For this review, take the finished solid that the model builds, in its own axes (mm). A direction names the side the tool comes from. Coordinates: 2 decimals unless noted, no trailing zeros. Write each loop counter-clockwise with the first axis right and the second up, starting at its lowest first coordinate (ties: lowest second). Pieces come first, ordered by that corner, then holes.
Autodesk Inventor part; units mm, degrees
ref_plane "YZ Plane" through (0, 0, 0) normal (1, 0, 0) x (0, 1, 0)
ref_plane "XZ Plane" through (0, 0, 0) normal (0, 1, 0) x (-1, 0, 0)
ref_plane "XY Plane" through (0, 0, 0) normal (0, 0, 1) x (1, 0, 0)
sketch "Sketch1" plane through (0, 0, 0) normal (0, 0, 1) x (1, 0, 0)
  line L0 (-12.7, 0) -> (12.7, 0) construction
  line L1 (12.7, 0) -> (12.7, -57.15)
  line L2 (12.7, -57.15) -> (-12.7, -57.15)
  line L3 (-12.7, -57.15) -> (-12.7, 0) construction
  line L4 (-35.1269, 0) -> (-12.7, -11.9246) construction
  line L5 (-12.7, -11.9246) -> (-36.5492, -56.7783)
  line L6 (-36.5492, -56.7783) -> (-58.976, -44.8537)
  line L7 (-58.976, -44.8537) -> (-35.1269, 0)
  line L8 (-23.9134, -5.9623) -> (-47.7626, -50.816) construction
  line L9 (-35.1269, 0) -> (12.7, 0)
  line L10 (-12.7, -11.9246) -> (-12.7, -57.15)
  point P0 (0, 0)
  point P1 (0, 0)
  point P2 (-29.8757, -17.1757)
  point P3 (-41.8003, -39.6026)
  point P4 (0, -12.7)
  point P5 (0, -38.1)
  dimension "d0" = 25.4
  dimension "d1" = 25.4
  dimension "d2" = 28
  dimension "d3" = 50.8
  dimension "d4" = 25.4
  dimension "d5" = 12.7
  dimension "d6" = 25.4
  dimension "d7" = 12.7
  dimension "d8" = 57.15
extrude "Extrusion1" add sketch "Sketch1" against normal blind 6.35
hole "Hole1" at (-29.8757, -17.1757, 0) at (-41.8003, -39.6026, 0) at (0, -12.7, 0) at (0, -38.1, 0) direction (0, 0, -1) diameter 5.1054 end through all
sketch "Sketch2" plane through (0, 0, 0) normal (0, 0, 1) x (1, 0, 0)
  circle A0 centre (0, -12.7) radius 2.5527 construction
  circle A1 centre (-29.8757, -17.1757) radius 2.5527 construction
  circle A2 centre (-41.8003, -39.6026) radius 2.5527 construction
  circle A3 centre (0, -38.1) radius 2.5527 construction
  line L0 (-12.7, -57.15) -> (12.7, -57.15) construction
  line L1 (12.7, -57.15) -> (12.7, 0) construction
  line L2 (12.7, 0) -> (-35.1269, 0)
  line L3 (-35.1269, 0) -> (-58.976, -44.8537) construction
  line L4 (-58.976, -44.8537) -> (-36.5492, -56.7783) construction
  line L5 (-36.5492, -56.7783) -> (-12.7, -11.9246) construction
  line L6 (-12.7, -11.9246) -> (-12.7, -57.15) construction
  circle A4 centre (0, -12.7) radius 2.5527 construction
  circle A5 centre (-29.8757, -17.1757) radius 2.5527 construction
  circle A6 centre (-41.8003, -39.6026) radius 2.5527 construction
  circle A7 centre (0, -38.1) radius 2.5527 construction
  line L7 (12.7, 0) -> (12.7, -57.15) construction
  line L8 (12.7, -57.15) -> (-12.7, -57.15) construction
  line L9 (-12.7, -57.15) -> (-12.7, -11.9246) construction
  line L10 (-36.5492, -56.7783) -> (-58.976, -44.8537) construction
  line L11 (-58.976, -44.8537) -> (-35.1269, 0) construction
  line L12 (-35.1269, 0) -> (12.7, 0) construction
  circle A8 centre (-11.2134, 101.6) radius 14.2875 construction
  line L13 (12.7, 0) -> (-35.1269, 0) construction
  line L14 (-35.1269, 0) -> (-58.976, -44.8537) construction
  circle A9 centre (0, -12.7) radius 2.5527 construction
  circle A10 centre (-29.8757, -17.1757) radius 2.5527 construction
  circle A11 centre (-41.8003, -39.6026) radius 2.5527 construction
  circle A12 centre (0, -38.1) radius 2.5527 construction
  line L15 (12.7, 0) -> (12.7, -57.15) construction
  line L16 (12.7, -57.15) -> (-12.7, -57.15) construction
  line L17 (-12.7, -57.15) -> (-12.7, -11.9246) construction
  line L18 (-36.5492, -56.7783) -> (-58.976, -44.8537) construction
  line L19 (-58.976, -44.8537) -> (-35.1269, 0) construction
  line L20 (-35.1269, 0) -> (12.7, 0) construction
  line L21 (-35.1269, 0) -> (12.7, 0) construction
  line L22 (12.7, 0) -> (12.7, 122.2375)
  line L23 (12.7, 122.2375) -> (-35.1269, 122.2375)
  line L24 (-35.1269, 122.2375) -> (-35.1269, 0)
  line L25 (-12.7, -11.9246) -> (-36.5492, -56.7783)
  line L26 (-35.1269, 122.2375) -> (-31.8509, 122.2375)
  line L27 (-31.8509, 122.2375) -> (-31.8509, 80.9625)
  line L28 (-31.8509, 80.9625) -> (-35.1269, 80.9625)
  line L29 (-35.1269, 80.9625) -> (-35.1269, 122.2375)
  line L30 (-12.7, -11.9246) -> (-36.5492, -56.7783)
  point P0 (0, 0)
  point P1 (-11.2134, 0)
  point P2 (-11.2134, 0)
  point P3 (-11.2134, 115.8875)
  point P4 (-11.2134, 122.2375)
  point P5 (-11.2134, 87.3125)
  point P6 (-25.5009, 101.6)
  point P7 (-35.1269, 80.9625)
  dimension "d19" = 28.575
  dimension "d20" = 101.6
  dimension "d32" = 6.35
  dimension "d36" = 0
  dimension "d37" = 6.35
  dimension "d38" = 6.35
extrude "Extrusion2" add sketch "Sketch2" against normal up to surface (6.35 mm away)
fillet "Fillet1" radius 6.35 6 edges at (12.7, -57.15, -3.175) (-12.7, -57.15, -3.175) (-12.7, -11.9246, -3.175) (-36.5492, -56.7783, -3.175) (-58.976, -44.8537, -3.175) (-35.1269, 0, -3.175)
hole "Hole2" at (-11.2134, 101.6, 0) direction (0, 0, -1) diameter 28.575 end through all
fillet "Fillet2" radius 12.7 2 edges at (12.7, 122.2375, -3.175) (-35.1269, 122.2375, -3.175)
equation "\"d38\" = d32"
properties part number "CL6-001" material "Aluminum 6061"
Q1. Draft analysis for pull direction X (two halves, no side actions). For faces 4 (the cylindrical face through (10.89, -55.24, -3.22)), 5 (the cylindrical face through (-32.4, -16.8, -3.2)), 6 (the cylindrical face through (-35.31, 0.07, -3.22)), state which applies: +X half, -X half, draft (parallel to the pull), parting line (faces both ways), or undercut.
Ans:
face 4: +X half
face 5: undercut
face 6: -X half
Q2. Add section A-A (y = 101.6). State the section outline as (x, z) points, then the cut area to 3 significant figures.
Ans:
outline: (-35.13, -6.35) - (-25.5, -6.35) - (-25.5, 0) - (-35.13, 0) - close; (3.07, -6.35) - (12.7, -6.35) - (12.7, 0) - (3.07, 0) - close
area: 122 mm2
Q3. Add section B-B (z = -2.75). Give the number of separate pieces and of enclosed holes in the cut face, then the cut area to 3 significant figures.
Ans:
separate pieces: 1
enclosed holes: 5
area: 8,000 mm2
Q4. Add section C-C (y = 38.5). State the section outline as (x, z) points, then the cut area to 3 significant figures.
Ans:
outline: (-35.13, -6.35) - (12.7, -6.35) - (12.7, 0) - (-35.13, 0) - close
area: 304 mm2
Q5. Tool access review of faces 1 (the flat face through (-15, 34, -6.35)), 2 (the flat face through (-35.127, 56, -3)), 3 (the flat face through (-12.7, -44, -3)): name each direction out of +Z, -Z, +X, -X, +Y, -Y from which nothing blocks a thin tool from reaching the whole face with its end or side.
Ans:
face 1: -Z, +X, -X, +Y, -Y
face 2: +Z, -Z, -X, +Y
face 3: +Z, -Z, -Y
Q6. Clearance check with flat-ended pins moving along their axes: pin 1 Ø2 at (x, z) = (-44, -4) entering from +Y; pin 2 Ø1.9 at (y, z) = (-45, -4) entering from -X; pin 3 Ø4 at (x, y) = (-29.88, -17.18) entering from +Z. State where each tip first meets the part, or that it passes through.
Ans:
pin 1: stops at y = -14.81
pin 2: stops at x = -56.47
pin 3: passes through
Q7. Add section D-D (y = -46). State the section outline as (x, z) points, then the cut area to 3 significant figures.
Ans:
outline: (-55.5, -6.35) - (-30.82, -6.35) - (-30.82, 0) - (-55.5, 0) - close; (-12.7, -6.35) - (12.7, -6.35) - (12.7, 0) - (-12.7, 0) - close
area: 318 mm2
Q8. For probe 1 along X at (y, z) = (101.6, -2.75); probe 2 along X at (y, z) = (-38.1, -4.75) (3 decimals); probe 3 along X at (y, z) = (45, -1.75), list the stretches that pass through material, from the lowest coordinate up.
Ans:
probe 1: x = -35.13 to -25.5, 3.07 to 12.7
probe 2: x = -55.385 to -43.864, -39.737 to -26.618, -12.7 to -2.553, 2.553 to 12.7
probe 3: x = -35.13 to 12.7
